from build123d import *

# Parameters (mm, degrees)
CROQUIS1_W                  = 74
CROQUIS1_H                  = 59
SALIENTE_EXTRUIR1_DEPTH     = 25
VACIADO1_T                  = -2
VACIADO1_THICKNESS_2_FACE_W = 23
VACIADO1_THICKNESS_2_FACE_H = 55
VACIADO1_THICKNESS_2_DEPTH  = 0.8
CORTAR_EXTRUIR1_DEPTH       = 1.2


with BuildPart() as part:
    # Croquis1 → Saliente-Extruir1 (new body)
    with BuildSketch(Plane.XY):
        with Locations((627.712029931, -11.748201439)):
            Rectangle(CROQUIS1_W, CROQUIS1_H)
    extrude(amount=SALIENTE_EXTRUIR1_DEPTH)

    # Vaciado1
    vaciado1_openings = [part.faces().sort_by_distance(p)[0] for p in [
        (627.712029931, -11.748201439, 25),
    ]]
    offset(amount=VACIADO1_T, openings=vaciado1_openings, kind=Kind.INTERSECTION)

    # Vaciado1 thickness 2 face (on inner face of the shell) → Vaciado1 thickness 2 (cut)
    with BuildSketch(Plane(origin=(592.712029931, -11.748201439, 13.5), x_dir=(0, 0, -1), z_dir=(-1, 0, 0))):
        Rectangle(VACIADO1_THICKNESS_2_FACE_W, VACIADO1_THICKNESS_2_FACE_H)
    extrude(amount=VACIADO1_THICKNESS_2_DEPTH, mode=Mode.SUBTRACT)

    # Croquis2 → Cortar-Extruir1 (cut)
    with BuildSketch(Plane.ZY.offset(-590.712029931)):
        with BuildLine():
            Line((21.9, -7.072321113), (25, -7.072321113))
            Line((25, -7.072321113), (25, -16.172321113))
            Line((25, -16.172321113), (21.9, -16.172321113))
            ThreePointArc((21.9, -16.172321113), (21.192893219, -15.879427895), (20.9, -15.172321113))
            Line((20.9, -15.172321113), (20.9, -8.072321113))
            ThreePointArc((20.9, -8.072321113), (21.192893219, -7.365214332), (21.9, -7.072321113))
        make_face()
    extrude(amount=-CORTAR_EXTRUIR1_DEPTH, mode=Mode.SUBTRACT)


solid = part.part
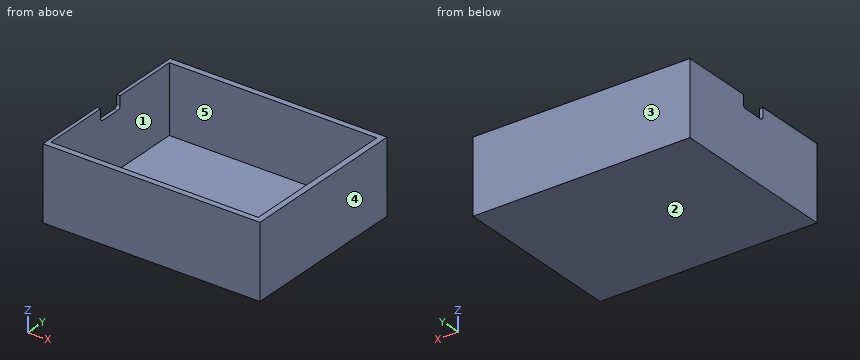
The model under review builds one solid part; all positions refer to its coordinate system, in mm. Face numbers are marked on the shaded views. A direction names the side the tool comes from. Coordinates: 2 decimals unless noted, no trailing zeros. Loops run counter-clockwise (first coordinate to the right, second up) from the corner with the lowest first, then second, coordinate; pieces in that order, holes last.
(1) Consider section A-A, the plane z = 15.5. Give the boundary of the cut face in (x, y).
Determined:
outline: (590.71, -41.25) - (664.71, -41.25) - (664.71, 17.75) - (590.71, 17.75) - close; hole (591.91, -39.25) - (662.71, -39.25) - (662.71, 15.75) - (591.91, 15.75) - close
(2) Tool access review of the marked faces 1 and 2: name each direction out of +Z, -Z, +X, -X, +Y, -Y from which nothing blocks a thin tool from reaching the whole face with its end or side.
Determined:
face 1: +Z
face 2: -Z, +X, -X, +Y, -Y
(3) Consider section D-D, the plane z = 23.5. Give the boundary of the cut face in (x, y), plus the area to 3 significant figures.
Determined:
outline: (590.71, -41.25) - (664.71, -41.25) - (664.71, 17.75) - (590.71, 17.75) - (590.71, -7.07) - (591.91, -7.07) - (591.91, 15.75) - (662.71, 15.75) - (662.71, -39.25) - (591.91, -39.25) - (591.91, -16.17) - (590.71, -16.17) - close
area: 461 mm2
(4) Consider section B-B, the plane x = 624.5. Give the boundary of the cut face in (y, z), plus the area to 3 significant figures.
Determined:
outline: (-41.25, 0) - (17.75, 0) - (17.75, 25) - (15.75, 25) - (15.75, 2) - (-39.25, 2) - (-39.25, 25) - (-41.25, 25) - close
area: 210 mm2
(5) Consider section C-C, the plane y = -12. Give the boundary of the cut face in (x, z).
Determined:
outline: (590.71, 0) - (664.71, 0) - (664.71, 25) - (662.71, 25) - (662.71, 2) - (591.91, 2) - (591.91, 20.9) - (590.71, 20.9) - close
(6) Draft analysis for pull direction X (two halves, no side actions). For the marked faces 3, 4 and 5, state which applies: +X half, -X half, draft (parallel to the pull), parting line (faces both ways), or undercut.
Determined:
face 3: draft
face 4: +X half
face 5: undercut
(7) Insertion check: P1, Ø4, axis at x = 652, y = -11, coming from the +Z side; P2, Ø0.6, axis at x = 591, y = -12.5, coming from the +Z side. Each pin has a flat end and moves straight along its axis. Give the tip position at first contact, or say it passes through.
Determined:
P1: stops at z = 2
P2: stops at z = 20.9
(8) Wall thickness on L1, parallel to Y at x = 640, z = 21.5; L2, parallel to X at y = -14.5, z = 7.25; L3, parallel to Z at x = 625, y = -22: over which ranges is each line inside the solid? List them lowest first.
Determined:
L1: y = -41.25 to -39.25, 15.75 to 17.75
L2: x = 590.71 to 591.91, 662.71 to 664.71
L3: z = 0 to 2
